Source: CAD feature listing. Evaluate the final solid. Frame: model axes, mm. Coordinates: 2 decimals unless noted, no trailing zeros. Write each loop counter-clockwise with the first axis right and the second up, starting at its lowest first coordinate (ties: lowest second). Pieces come first, ordered by that corner, then holes. Notation, with made-up numbers: (39.25, 23) - (95.25, 23) arc R15 cw to (95.25, 48) - close; hole circle Ø3 at (43.25, -8.75). An arc over 180 degrees is marked (long way). One line per question, with ' | ' between items. Start each with the question number.
Q1. Line query: line 1 (Z direction, x = 61, y = -0.5); line 2 (Y direction, x = 66.5, z = 6); line 3 (X direction, y = -7.75, z = 4.25). Output: solid intervals per line, ascending.
Q2. Contact query for flat-ended pins moving along their axis: P1, Ø6, axis at y = 7, z = 12, coming from the -X side; P2, Ø8, axis at x = 120.5, z = 7.5, coming from the +Y side; P3, Ø6, axis at x = 57, y = 4.5, coming from the -Z side. Output: stop coordinate, or through.
Q3. Cut plane A-A, the plane y = 0. Return loops of the section in (x, z), plus the area to 3 significant figures.
Q4. Cut plane B-B, the plane z = 5. Return loops of the section in (x, y), plus the area to 3 significant figures.
Q5. Cut plane D-D, the plane z = 12.5. Return loops of the section in (x, y).
Q6. Cut plane C-C, the plane x = 156. Return loops of the section in (y, z).
```python
from build123d import *

# Parameters (mm, degrees)
SKETCH1_R             = 15
BOSS_EXTRUDE1_DEPTH   = 10
BOSS_EXTRUDE1_2_DEPTH = 10
SKETCH2_R             = 15
BOSS_EXTRUDE2_DEPTH   = 10
BOSS_EXTRUDE2_TAPER   = 20
BOSS_EXTRUDE3_DEPTH   = 5
BOSS_EXTRUDE4_DEPTH   = 5
SKETCH13_R            = 4
CUT_EXTRUDE1_DEPTH    = 20
BOSS_EXTRUDE7_START   = 2.5
SKETCH14_R            = 15
SKETCH14_R_2          = 4
BOSS_EXTRUDE7_DEPTH   = 2.5
ECHELLE1_SCALE        = 0.6


with BuildPart() as part:
    # Sketch1 → Boss-Extrude1 (new body)
    with BuildSketch(Plane.XY):
        Circle(SKETCH1_R)
    extrude(amount=BOSS_EXTRUDE1_DEPTH)

    # Sketch2 → Boss-Extrude2 (add)
    with BuildSketch(Plane.XY.offset(10)):
        Circle(SKETCH2_R)
    extrude(amount=BOSS_EXTRUDE2_DEPTH, taper=BOSS_EXTRUDE2_TAPER)



with BuildPart() as body_2:
    # Sketch1 → Boss-Extrude1 2 (new body)
    with BuildSketch(Plane.XY):
        with Locations((215, 0)):
            Circle(SKETCH1_R)
    extrude(amount=BOSS_EXTRUDE1_2_DEPTH)


with BuildPart() as part_1:
    add(part.part)

    add(body_2.part)  # Boss-Extrude3 merges body 2
    # Sketch5 → Boss-Extrude3 (add)
    with BuildSketch(Plane.XY):
        with BuildLine():
            Line((203.819660113, 10), (11.180339887, 10))
            ThreePointArc((11.180339887, 10), (14.012585384, 5.352331347), (15, 0))
            ThreePointArc((15, 0), (14.012585384, -5.352331347), (11.180339887, -10))
            Line((11.180339887, -10), (203.819660113, -10))
            ThreePointArc((203.819660113, -10), (200, 0), (203.819660113, 10))
        make_face()
    extrude(amount=BOSS_EXTRUDE3_DEPTH)

    # Sketch6 → Boss-Extrude4 (add)
    with BuildSketch(Plane.XY.offset(5)):
        with BuildLine():
            ThreePointArc((15, 0), (14.947457842, -1.254393904), (14.790199458, -2.5))
            ThreePointArc((14.790199458, -2.5), (13.515906498, -6.505403256), (11.180339887, -10))
            Line((11.180339887, -10), (203.819660113, -10))
            ThreePointArc((203.819660113, -10), (200, 0), (203.819660113, 10))
            Line((203.819660113, 10), (11.180339887, 10))
            ThreePointArc((11.180339887, 10), (13.515906498, 6.505403256), (14.790199458, 2.5))
            ThreePointArc((14.790199458, 2.5), (14.947457842, 1.254393904), (15, 0))
        make_face()
    extrude(amount=BOSS_EXTRUDE4_DEPTH)

    # Sketch13 → Cut-Extrude1 (cut)
    with BuildSketch(Plane(origin=(0, 0, 0), x_dir=(-1, 0, 0), z_dir=(0, 0, -1))):
        with Locations((-215, 0)):
            Circle(SKETCH13_R)
        Circle(SKETCH13_R)
    extrude(amount=-CUT_EXTRUDE1_DEPTH, mode=Mode.SUBTRACT)

    # Sketch14 → Boss-Extrude7 (add)
    with BuildSketch(Plane(origin=(0, 0, 0), x_dir=(-1, 0, 0), z_dir=(0, 0, -1)).offset(BOSS_EXTRUDE7_START)):
        Circle(SKETCH14_R)
        Circle(SKETCH14_R_2, mode=Mode.SUBTRACT)
    extrude(amount=-BOSS_EXTRUDE7_DEPTH)


with BuildPart() as part_2:
    # Echelle1: scaled about (95.047310585, 0, 5.648530127)
    add(part_1.part.scale(ECHELLE1_SCALE).moved(Location((38.018924234, 0, 2.259412051))))


solid = part_2.part
```
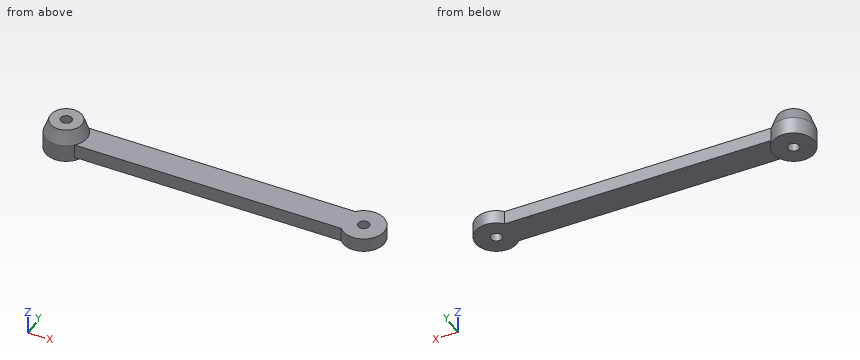
Reply:
1) line 1: z = 2.26 to 8.26 | line 2: y = -6 to 6 | line 3: x = 33.44 to 42.59, 162.44 to 171.59
2) P1: stops at x = 31.11 | P2: stops at y = 6 | P3: stops at z = 2.26
3) outline: (29.02, 0.76) - (35.62, 0.76) - (35.62, 14.26) - (31.2, 14.26) - (29.02, 8.26) - close; (40.42, 0.76) - (47.02, 0.76) - (47.02, 2.26) - (164.62, 2.26) - (164.62, 8.26) - (47.02, 8.26) - (44.84, 14.26) - (40.42, 14.26) - close; (169.42, 2.26) - (176.02, 2.26) - (176.02, 8.26) - (169.42, 8.26) - close | area: 910 mm^2
4) outline: (44.73, -6) - (160.31, -6) arc R9 ccw (long way) to (160.31, 6) - (44.73, 6) arc R9 ccw (long way) to start; hole circle Ø4.8 at (38.02, 0); hole circle Ø4.8 at (167.02, 0) | area: 1,820 mm^2
5) outline: circle Ø14.91 at (38.02, 0); hole circle Ø4.8 at (38.02, 0)
6) outline: (-6, 2.26) - (6, 2.26) - (6, 8.26) - (-6, 8.26) - close
